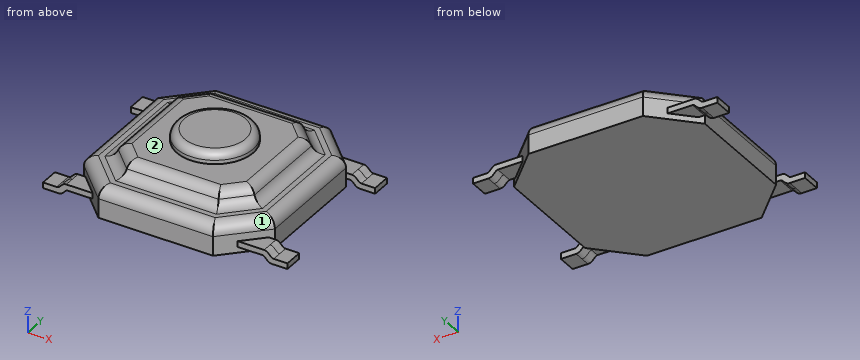
from build123d import *

# Parameters (mm, degrees)
BOSS_EXTRUDE1_DEPTH = 0.8
BOSS_EXTRUDE2_DEPTH = 0.4
SKETCH3_R           = 1
BOSS_EXTRUDE3_DEPTH = 0.3
FILLET1_R           = 0.3
FILLET2_R           = 0.3
FILLET3_R           = 0.3
FILLET4_R           = 0.2
BOSS_EXTRUDE4_DEPTH = 0.25


with BuildPart() as part:
    # Sketch1 → Boss-Extrude1 (new body)
    with BuildSketch(Plane.XY):
        Polygon((-1.5, 2.5), (1.5, 2.5), (2.5, 1.5), (2.5, -1.5), (1.5, -2.5), (-1.5, -2.5), (-2.5, -1.5), (-2.5, 1.5), align=None)
    extrude(amount=BOSS_EXTRUDE1_DEPTH)

    # Sketch2 → Boss-Extrude2 (add)
    with BuildSketch(Plane.XY.offset(0.8)):
        Polygon((-1.210050506, 1.8), (-1.8, 1.210050506), (-1.8, -1.210050506), (-1.210050506, -1.8), (1.210050506, -1.8), (1.8, -1.210050506), (1.8, 1.210050506), (1.210050506, 1.8), align=None)
    extrude(amount=BOSS_EXTRUDE2_DEPTH)

    # Sketch3 → Boss-Extrude3 (add)
    with BuildSketch(Plane.XY.offset(1.2)):
        Circle(SKETCH3_R)
    extrude(amount=BOSS_EXTRUDE3_DEPTH)

    # Fillet1
    fillet1_edges = [part.edges().sort_by_distance(p)[0] for p in [
        (1.505025253, 1.505025253, 1.2),
        (0, 1.8, 1.2),
        (-1.505025253, 1.505025253, 1.2),
        (-1.8, 0, 1.2),
        (-1.505025253, -1.505025253, 1.2),
        (0, -1.8, 1.2),
        (1.505025253, -1.505025253, 1.2),
        (1.8, 0, 1.2),
    ]]
    fillet(fillet1_edges, radius=FILLET1_R)

    # Fillet2
    fillet2_edges = [part.edges().sort_by_distance(p)[0] for p in [
        (-2, 2, 0.8),
        (-2.5, 0, 0.8),
        (-2, -2, 0.8),
        (0, -2.5, 0.8),
        (2, -2, 0.8),
        (2.5, 0, 0.8),
        (2, 2, 0.8),
        (0, 2.5, 0.8),
    ]]
    fillet(fillet2_edges, radius=FILLET2_R)

    # Fillet3
    fillet3_edges = [part.edges().sort_by_distance(p)[0] for p in [
        (0, -1.8, 0.8),
        (1.505025253, -1.505025253, 0.8),
        (1.8, 0, 0.8),
        (1.505025253, 1.505025253, 0.8),
        (0, 1.8, 0.8),
        (-1.505025253, 1.505025253, 0.8),
        (-1.8, 0, 0.8),
        (-1.505025253, -1.505025253, 0.8),
    ]]
    fillet(fillet3_edges, radius=FILLET3_R)

    # Fillet4
    fillet4_edges = [part.edges().sort_by_distance(p)[0] for p in [
        (-1, 0, 1.5),
    ]]
    fillet(fillet4_edges, radius=FILLET4_R)

    # Sketch4 → Boss-Extrude4 (add, symmetric)
    with BuildSketch(Plane(origin=(0, 1.85, 0), x_dir=(1, 0, 0), z_dir=(0, 1, 0))):
        with BuildLine():
            Line((0, -0.15), (-2.55, -0.15))
            add(Edge.make_bspline(
                [(-2.8, 0), (-2.662431202, 0), (-2.630462892, -0.15), (-2.55, -0.15)],
                knots=[0, 0, 0, 0, 1, 1, 1, 1], degree=3))
            Line((-2.8, 0), (-3.2, 0))
            Line((-3.2, 0), (-3.2, -0.15))
            Line((-3.2, -0.15), (-2.841547595, -0.15))
            add(Edge.make_bspline(
                [(-2.591547595, -0.3), (-2.713318055, -0.3), (-2.744365063, -0.15), (-2.841547595, -0.15)],
                knots=[0, 0, 0, 0, 1, 1, 1, 1], degree=3))
            Line((-2.591547595, -0.3), (0, -0.3))
            Line((0, -0.3), (2.591547595, -0.3))
            add(Edge.make_bspline(
                [(2.591547595, -0.3), (2.713318055, -0.3), (2.744365063, -0.15), (2.841547595, -0.15)],
                knots=[0, 0, 0, 0, 1, 1, 1, 1], degree=3))
            Line((2.841547595, -0.15), (3.2, -0.15))
            Line((3.2, -0.15), (3.2, 0))
            Line((3.2, 0), (2.8, 0))
            add(Edge.make_bspline(
                [(2.8, 0), (2.662431202, 0), (2.630462892, -0.15), (2.55, -0.15)],
                knots=[0, 0, 0, 0, 1, 1, 1, 1], degree=3))
            Line((2.55, -0.15), (0, -0.15))
        make_face()
    boss_extrude4 = extrude(amount=BOSS_EXTRUDE4_DEPTH, both=True)

    # Mirror1: Boss-Extrude4 across plane
    add(boss_extrude4.mirror(Plane.ZX))


solid = part.part
For this review, take the finished solid that the model builds, in its own axes (mm). Face numbers are marked on the shaded views. A direction names the side the tool comes from. Round coordinates to 2 decimals unless told otherwise and drop trailing zeros. Loops run counter-clockwise (first coordinate to the right, second up) from the corner with the lowest first, then second, coordinate; pieces in that order, holes last. Notation, with made-up numbers: (78.25, -22) - (107.25, -22) arc R26 cw to (107.25, 11) - close; hole circle Ø4 at (45, 39). An arc over 180 degrees is marked (long way). Use one line per item in the form item = value.
1) Tool access review of the marked faces 1 and 2: name each direction out of +Z, -Z, +X, -X, +Y, -Y from which nothing blocks a thin tool from reaching the whole face with its end or side.
Solutions:
face_1 = +Z, +X, -Y
face_2 = +Z
2) Wall thickness on probe 1 along Z at (x, y) = (1.25, 1.3); probe 2 along Z at (x, y) = (-0.75, 2.05); probe 3 along X at (y, z) = (-0.8, 0.7): over which ranges is each line inside the solid? List them lowest first.
Solutions:
probe_1 = 0 to 1.2
probe_2 = 0 to 0.8
probe_3 = -2.42 to 2.42
3) Clearance check with flat-ended pins moving along their axes: P1, Ø0.6, axis at x = 2.5, y = -2, coming from the +Z side; P2, Ø0.6, axis at y = -0.5, z = 0, coming from the -X side; P3, Ø0.6, axis at x = 2.5, y = 1.5, coming from the +Z side. State where each tip first meets the part, or that it passes through.
Solutions:
P1 = 0.3
P2 = -2.5
P3 = 0.8
4) We need section A-A on z = 0.65. Write out the cut boundary in (x, y).
Solutions:
outline = (-2.46, -1.48) - (-1.48, -2.46) - (1.48, -2.46) - (2.46, -1.48) - (2.46, 1.48) - (1.48, 2.46) - (-1.48, 2.46) - (-2.46, 1.48) - close
